Read the model definition and answer for the solid it produces. Units are mm, in the model's axes. A direction names the side the tool comes from. Give positions to 0.01 mm unless a question says otherwise; leave off trailing zeros. Order: outer loops, then holes, each group sorted by start corner. A loop starts at its lowest first (then second) coordinate and runs counter-clockwise, first axis right, second up. Notation, with made-up numbers: M 63.5,67 L 98.5,67 A11 cw 98.5,80 Z; hole C -29.75,-9.5 d8. An arc over 180 degrees is marked long. One line per item, written item: value.
from build123d import *

# Parameters (mm, degrees)
F1_DEPTH = 4.7625
F3_DEPTH = 46.0375


with BuildPart() as f1:
    # F0 (on Front) → F1 (new body)
    with BuildSketch(Plane.XZ):
        Polygon((457.2, 584.2), (-177.8, 584.2), (-177.8, 0), (0, 0), (0, -949.325), (457.2, -949.325), align=None)
        Polygon((50.8, -898.525), (50.8, 50.8), (-127, 50.8), (-127, 533.4), (406.4, 533.4), (406.4, -898.525), align=None, mode=Mode.SUBTRACT)
    extrude(amount=F1_DEPTH)

    # F2 (on face) → F3 (join)
    with BuildSketch(Plane(origin=(0, 0, 0), x_dir=(-1, 0, 0), z_dir=(0, 1, 0))):
        Polygon((177.8, 584.2), (-457.2, 584.2), (-457.2, -949.325), (0, -949.325), (0, 0), (177.8, 0), align=None)
        Polygon((-4.7625, -944.5625), (-452.4375, -944.5625), (-452.4375, 579.4375), (173.0375, 579.4375), (173.0375, 4.7625), (-4.7625, 4.7625), align=None, mode=Mode.SUBTRACT)
    extrude(amount=F3_DEPTH)


solid = f1.part
1) Consider probe 1 along Z at (x, y) = (119, 12.5) (1 decimal); probe 2 along X at (y, z) = (-1, 516); probe 3 along X at (y, z) = (-1.5, -269). Determine where each line is inside the solid, lowest interval first.
Reported:
probe 1: z = -949.3 to -944.6, 579.4 to 584.2
probe 2: x = -177.8 to -127, 406.4 to 457.2
probe 3: x = 0 to 50.8, 406.4 to 457.2
2) Each of these flat-tipped pins is pushed along its axis until it touches: pin 1 Ø1.5 at (y, z) = (4.5, -244.5) entering from -X; pin 2 Ø1 at (x, y) = (-16.5, 6) entering from -Z. Where does it stop, or does it pass through?
Reported:
pin 1: stops at x = 0
pin 2: stops at z = 0
3) Find section A-A, the plane x = 261.5. Write down the section's boundary in (y, z) (1 decimal).
Reported:
outline: M -4.8,-949.3 L 46,-949.3 L 46,-944.6 L 0,-944.6 L 0,-898.5 L -4.8,-898.5 Z; M -4.8,533.4 L 0,533.4 L 0,579.4 L 46,579.4 L 46,584.2 L -4.8,584.2 Z
4) Which of the six approach directions +Z, -Z, +X, -X, +Y, -Y give full straight-line access (tool end or side, diameter ignored) to faces 5 (the face through (-85, 23, 4.762)), 6 (the face through (457.2, 20, -172)), 7 (the face through (-88, 20, 0))?
Reported:
face 5: +Y
face 6: +Z, -Z, +X, +Y, -Y
face 7: -Z, -X, +Y, -Y
5) Determine the mould class of faces 1 (the face through (225, 23, -944.562)), 2 (the face through (135, 20, 584.2)), 3 (the face through (0, 20, -481)), 4 (the face through (46, 0, -123)) for opening direction Z: +Z half, -Z half, draft (parallel to the pull), parting line (faces both ways), or undercut.
Reported:
face 1: undercut
face 2: +Z half
face 3: draft
face 4: undercut
6) Find section B-B, the plane z = -88. Write down the section's boundary in (x, y).
Reported:
outline: M 0,-4.76 L 50.8,-4.76 L 50.8,0 L 4.76,0 L 4.76,46.04 L 0,46.04 Z; M 406.4,-4.76 L 457.2,-4.76 L 457.2,46.04 L 452.44,46.04 L 452.44,0 L 406.4,0 Z
7) Find section C-C, the plane y = 19. Write down the section's boundary in (x, z) (1 decimal), plus the area to 3 significant figures.
Reported:
outline: M -177.8,0 L 0,0 L 0,-949.3 L 457.2,-949.3 L 457.2,584.2 L -177.8,584.2 Z; hole M -173,4.8 L 4.8,4.8 L 4.8,-944.6 L 452.4,-944.6 L 452.4,579.4 L -173,579.4 Z
area: 20,600 mm^2
